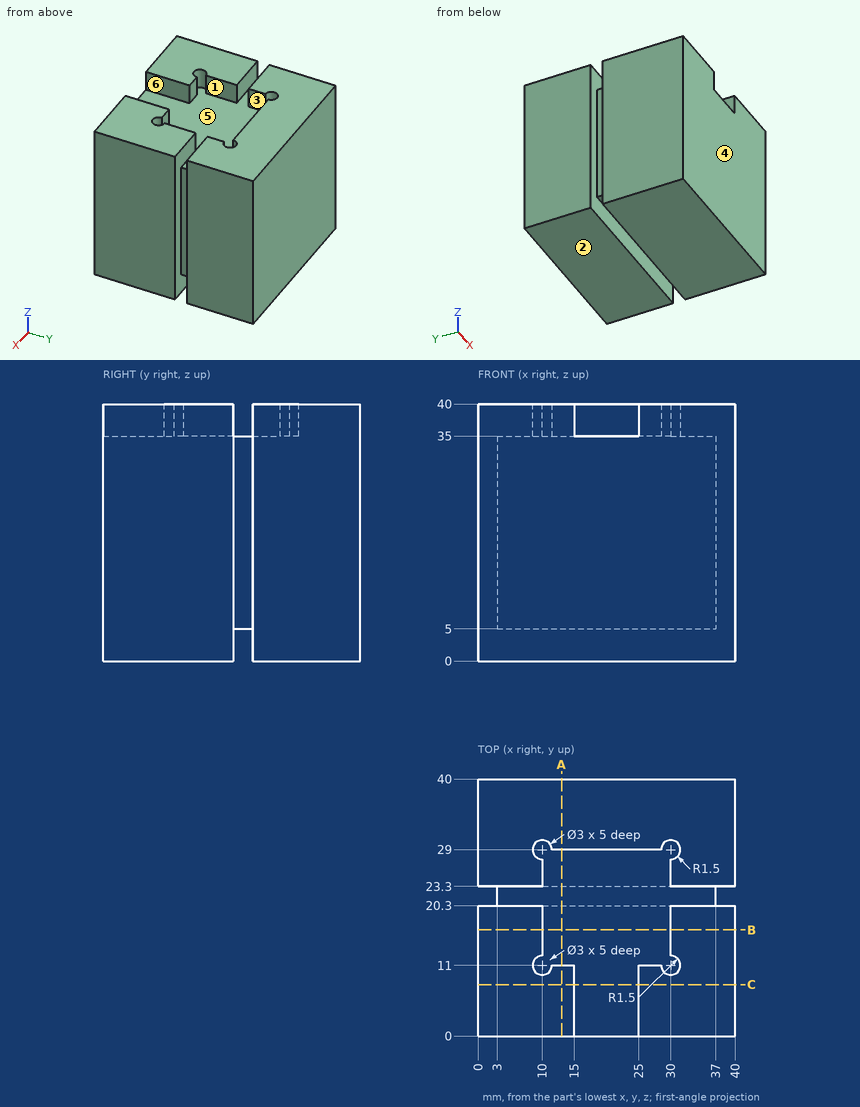
Could you check a few things on this drawing? It's one solid part, dimensions in mm from its lowest x, y, z. A direction names the side the tool comes from. Round coordinates to 2 decimals unless told otherwise and drop trailing zeros. Loops run counter-clockwise (first coordinate to the right, second up) from the corner with the lowest first, then second, coordinate; pieces in that order, holes last.
Q1. Thinking about a two-plate mould opening in Y: for the marked faces 3, 4, 5 and 6, which applies, pulls with the +Y half, pulls with the -Y half, needs draft (parallel to the pull), parting line crosses it, or undercut?
Q2. I want a section at A-A (x = 13). Write out the boundary of the cut face in (y, z).
Q3. I want a section at B-B (y = 16.5). Write out the boundary of the cut face in (x, z), and give its area (3 significant figures).
Q4. I want a section at C-C (y = 8). Write out the boundary of the cut face in (x, z).
Q5. Please list where these lines run through material, in increasing order: L1, parallel to Y at x = 19, z = 3.5; L2, parallel to Z at x = 19, y = 14; L3, parallel to Z at x = 21, y = 23.
Q6. For P1, Ø0.9, axis at y = 22, z = 16.5, coming from the -X side, with a flat end and sliding along its axis, tell me the tip position at first contact or that it passes through.
Q7. On a 3-axis mill with a long thin cutter (end or side, diameter ignored), from which of +Z, -Z, +X, -X, +Y, -Y can I reach the whole of each face in a straight line? I mean the marked faces 1 and 2. Say none if no direction works.
Answer below:
1. face 3: undercut
1. face 4: pulls with the -Y half
1. face 5: undercut
1. face 6: needs draft
2. outline: (0, 0) - (20.3, 0) - (20.3, 5) - (23.3, 5) - (23.3, 0) - (40, 0) - (40, 40) - (29, 40) - (29, 35) - (11, 35) - (11, 40) - (0, 40) - close
3. outline: (0, 0) - (40, 0) - (40, 40) - (30, 40) - (30, 35) - (10, 35) - (10, 40) - (0, 40) - close
3. area: 1,500 mm2
4. outline: (0, 0) - (40, 0) - (40, 40) - (25, 40) - (25, 35) - (15, 35) - (15, 40) - (0, 40) - close
5. L1: y = 0 to 20.3, 23.3 to 40
5. L2: z = 0 to 35
5. L3: z = 5 to 35
6. P1: stops at x = 3
7. face 1: +Z
7. face 2: -Z, +X, -X, +Y, -Y
